For this review, use the dimensioned drawing (mm, ordinates from the lowest corner) and the shaded views. A direction names the side the tool comes from. Round coordinates to 2 decimals unless told otherwise and drop trailing zeros. Loops run counter-clockwise (first coordinate to the right, second up) from the corner with the lowest first, then second, coordinate; pieces in that order, holes last. Notation, with made-up numbers: (-31.75, -34.75) - (-25.75, -34.75) arc R31 ccw to (-25.75, 2.25) - close; hole circle Ø9 at (-12, 82.5). An arc over 180 degrees is marked (long way). One line per question, with ' | ' between items. Start each with the question number.
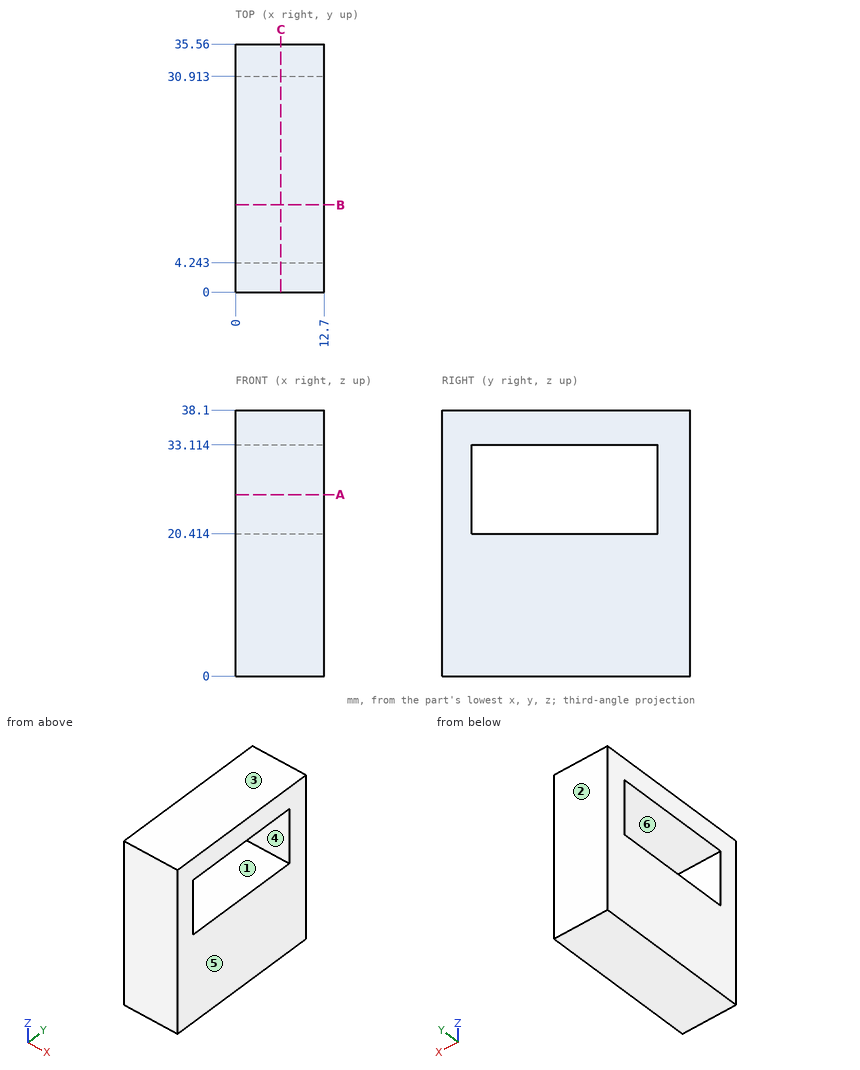
1. Take a section at C-C, the plane x = 6.5. Give the boundary of the cut face in (y, z).
2. Take a section at A-A, the plane z = 26. Give the boundary of the cut face in (x, y).
3. To check wall thickness, follow line 1 along Z through (x, y) = (11.5, 21); line 2 along Y through (x, z) = (4, 30.5). State the ranges of each line that lie inside material, in increasing order.
4. Machinability: for the marked faces 5 and 6, which of the approach directions +Z, -Z, +X, -X, +Y, -Y give a long, thin tool a straight path to every point of the face, cutting with its end or side? Answer none if there is none.
5. The part is to be moulded in two halves that separate along Y. For the marked faces 1, 2, 3 and 4, say which applies: pulls with the +Y half, pulls with the -Y half, needs draft (parallel to the pull), parting line crosses it, or undercut.
6. Take a section at B-B, the plane y = 12.5. Give the boundary of the cut face in (x, z).
Answer list:
1) outline: (0, 0) - (35.56, 0) - (35.56, 38.1) - (0, 38.1) - close; hole (4.24, 20.41) - (30.91, 20.41) - (30.91, 33.11) - (4.24, 33.11) - close
2) outline: (0, 0) - (12.7, 0) - (12.7, 4.24) - (0, 4.24) - close; (0, 30.91) - (12.7, 30.91) - (12.7, 35.56) - (0, 35.56) - close
3) line 1: z = 0 to 20.41, 33.11 to 38.1 | line 2: y = 0 to 4.24, 30.91 to 35.56
4) face 5: +Z, -Z, +X, +Y, -Y | face 6: +X, -X
5) face 1: undercut | face 2: pulls with the +Y half | face 3: needs draft | face 4: undercut
6) outline: (0, 0) - (12.7, 0) - (12.7, 20.41) - (0, 20.41) - close; (0, 33.11) - (12.7, 33.11) - (12.7, 38.1) - (0, 38.1) - close
